from build123d import *

# Parameters (mm, degrees)
BOSS_EXTRUDE1_DEPTH = 18.25625
FILLET1_R           = 3.3782


with BuildPart() as part:
    # Sketch3 → Boss-Extrude1 (new body)
    with BuildSketch(Plane(origin=(0, 0, 0), x_dir=(1, 0, 0), z_dir=(0, 1, 0))):
        with BuildLine():
            Line((469.9, -484.145858865), (469.9, -469.9))
            Line((469.9, -469.9), (404.8125, -404.8125))
            Line((404.8125, -404.8125), (395.2875, -404.8125))
            Line((395.2875, -404.8125), (395.2875, -464.068909047))
            ThreePointArc((395.2875, -464.068909047), (0, -609.6), (-395.2875, -464.068909047))
            Line((-395.2875, -464.068909047), (-395.2875, -404.8125))
            Line((-395.2875, -404.8125), (-404.8125, -404.8125))
            Line((-404.8125, -404.8125), (-469.9, -469.9))
            Line((-469.9, -469.9), (-469.9, -484.145858865))
            ThreePointArc((-469.9, -484.145858865), (0, -674.6875), (469.9, -484.145858865))
        make_face()
    extrude(amount=BOSS_EXTRUDE1_DEPTH)

    # Fillet1
    fillet1_edges = [part.edges().sort_by_distance(p)[0] for p in [
        (-395.2875, 9.128125, 464.068909047),
        (395.2875, 9.128125, 464.068909047),
    ]]
    fillet(fillet1_edges, radius=FILLET1_R)


solid = part.part
Design review of the part built by this model. Coordinates are the model's own, in mm. A direction names the side the tool comes from. Give positions to 0.01 mm unless a question says otherwise; leave off trailing zeros. Loops run counter-clockwise (first coordinate to the right, second up) from the corner with the lowest first, then second, coordinate; pieces in that order, holes last. Notation, with made-up numbers: M -16,7 L -4,7 A25 ccw -4,41 Z; hole C 73.25,73.25 d3. An arc over 180 degrees is marked long. Answer as a JSON object with one key per item and string values.
Item 1: We need section D-D (x = -347). State the section outline as (y, z) points.
Output values:
{"outline": "M 0,501.2 L 18.26,501.2 L 18.26,578.61 L 0,578.61 Z"}
Item 2: Mouldability with a two-part tool opening along X and no side actions: class faces 1 (the face through (-437, 9, 437)), 2 (the face through (438, 9, 438)), 3 (the face through (-2, 18.256, 619)), 4 (the face through (6, 9, 609.57)) as pulls with the +X half, pulls with the -X half, needs draft (parallel to the pull), parting line crosses it, or undercut.
Output values:
{"face 1": "pulls with the -X half", "face 2": "pulls with the +X half", "face 3": "needs draft", "face 4": "undercut"}
Item 3: Wall thickness on line 1 along X through (y, z) = (4.75, 451); line 2 along X through (y, z) = (8, 526.5); line 3 along Z through (x, y) = (-53, 9.75): over which ranges is each line inside the solid? List them lowest first.
Output values:
{"line 1": "x = -451 to -395.29, 395.29 to 451", "line 2": "x = -421.9 to -307.26, 307.26 to 421.9", "line 3": "z = 607.29 to 672.6"}
Item 4: For P1, Ø9, axis at y = 6.5, z = 446.5, coming from the +X side; P2, Ø5, axis at y = 14, z = 597, coming from the -X side; P3, Ø2, axis at x = -117, y = 2, coming from the -Z side, all flat-tipped, find the tip position at first contact; note any pin that passes through.
Output values:
{"P1": "stops at x = 451", "P2": "stops at x = -319.02", "P3": "stops at z = 598.07"}
Item 5: Machinability: for faces 5 (the face through (-395.288, 9, 434)), 6 (the face through (-2, 0, 619)), which of the approach directions +Z, -Z, +X, -X, +Y, -Y give a long, thin tool a straight path to every point of the face, cutting with its end or side? Answer none if there is none.
Output values:
{"face 5": "-Z, +Y, -Y", "face 6": "+Z, -Z, +X, -X, -Y"}
Item 6: We need section C-C (z = 508). State the section outline as (x, y) points, and give its area (3 significant figures).
Output values:
{"outline": "M -444,0 L -336.97,0 L -336.97,18.26 L -444,18.26 Z; M 336.97,0 L 444,0 L 444,18.26 L 336.97,18.26 Z", "area": "3,910 mm2"}
Item 7: We need section B-B (y = 12). State the section outline as (x, z) points (1 decimal), and give its area (3 significant figures).
Output values:
{"outline": "M -469.9,469.9 L -404.8,404.8 L -395.3,404.8 L -395.3,462.5 A3.4 cw -394.1,465.1 A609.6 cw 394.1,465.1 A3.4 cw 395.3,462.5 L 395.3,404.8 L 404.8,404.8 L 469.9,469.9 L 469.9,484.1 A674.7 ccw -469.9,484.1 Z", "area": "68,000 mm2"}
Item 8: We need section A-A (z = 572). State the section outline as (x, y) points, and give its area (3 significant figures).
Output values:
{"outline": "M -357.8,0 L -210.78,0 L -210.78,18.26 L -357.8,18.26 Z; M 210.78,0 L 357.8,0 L 357.8,18.26 L 210.78,18.26 Z", "area": "5,370 mm2"}
